Geometry check sheet. Reference: the model listing, model coordinates, mm. Round coordinates to 2 decimals unless told otherwise and drop trailing zeros. Write each loop counter-clockwise with the first axis right and the second up, starting at its lowest first coordinate (ties: lowest second). Pieces come first, ordered by that corner, then holes. Notation, with made-up numbers: M 22,69.5 L 59,69.5 A27 cw 59,98.5 Z; hole C -5,64 d9. An arc over 180 degrees is marked long. Use a Markdown table: item, result.
Autodesk Inventor part; units mm, degrees
ref_plane "YZ Plane" through (0, 0, 0) normal (1, 0, 0) x (0, 1, 0)
ref_plane "XZ Plane" through (0, 0, 0) normal (0, 1, 0) x (-1, 0, 0)
ref_plane "XY Plane" through (0, 0, 0) normal (0, 0, 1) x (1, 0, 0)
sketch "Szkic1" plane through (0, 0, 0) normal (0, 0, 1) x (1, 0, 0)
  line L0 (-475, -290) -> (475, -290)
  line L1 (475, -290) -> (475, 290)
  line L2 (475, 290) -> (-475, 290)
  line L3 (-475, 290) -> (-475, -290)
  line L4 (-475, -290) -> (475, 290) construction
  line L5 (475, -290) -> (-475, 290) construction
  point P0 (0, 0)
  dimension "d0" = 950
  dimension "d1" = 580
extrude "Wyciągnięcie proste1" add sketch "Szkic1" along normal blind 20
sketch "Szkic2" plane through (0, 0, 20) normal (0, 0, 1) x (1, 0, 0)
  line L0 (-475, -290) -> (475, -290)
  line L1 (475, -290) -> (475, 290)
  line L2 (475, 290) -> (-475, 290)
  line L3 (-475, 290) -> (-475, -290)
  line L4 (-475, -290) -> (475, -290)
  line L5 (-475, -290) -> (-375, -290)
  line L6 (-475, -290) -> (-375, -290) construction
  line L7 (-375, -290) -> (-375, 290)
  line L8 (-375, -290) -> (-375, -190)
  circle A0 centre (-375, -190) radius 10
  point P0 (0, 0)
  dimension "d4" = 100
  dimension "d5" = 0
  dimension "d6" = 100
  dimension "d7" = 20
extrude "Wyciągnięcie proste2" cut sketch "Szkic2" against normal up to next contours A0 L7 | L7 A0
pattern_linear "Szyk prostokątny1" count 5 spacing 100 along (0, 1, 0) count 9 spacing 94 along (1, 0, 0) of "Wyciągnięcie proste2"
properties part number "Sklejka stołu"
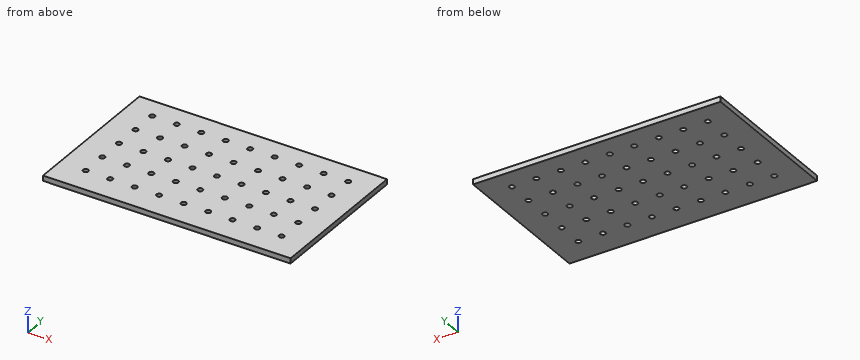
Item 1: Material ranges on line 1 along Y through (x, z) = (377, 7.25); line 2 along Y through (x, z) = (369, 12.5), recorded low to high. Write a range as from..to.
Outcome:
| item | result |
|---|---|
| line 1 | y = -290..-200, -180..-100, -80..0, 20..100, 120..200, 220..290 |
| line 2 | y = -290..-196, -184..-96, -84..4, 16..104, 116..204, 216..290 |
Item 2: Go/stop test with a flat-tipped pin: pin 1 (12 mm diameter, centred on x = -281, y = -90, fed in from +Z). Record where the tip stops, or that it passes through.
Outcome:
| item | result |
|---|---|
| pin 1 | passes through |
Item 3: Cross-section at B-B, the plane z = 7.25. Count the separate pieces of the cut face and the enclosed holes in it, and give its area (3 significant figures).
Outcome:
| item | result |
|---|---|
| separate pieces | 1 |
| enclosed holes | 45 |
| area | 537,000 mm2 |
Item 4: Cross-section at A-A, the plane x = -187. Record the cut outline in (y, z), and give its area (3 significant figures).
Outcome:
| item | result |
|---|---|
| outline | M -290,0 L -200,0 L -200,20 L -290,20 Z; M -180,0 L -100,0 L -100,20 L -180,20 Z; M -80,0 L 0,0 L 0,20 L -80,20 Z; M 20,0 L 100,0 L 100,20 L 20,20 Z; M 120,0 L 200,0 L 200,20 L 120,20 Z; M 220,0 L 290,0 L 290,20 L 220,20 Z |
| area | 9,600 mm2 |
